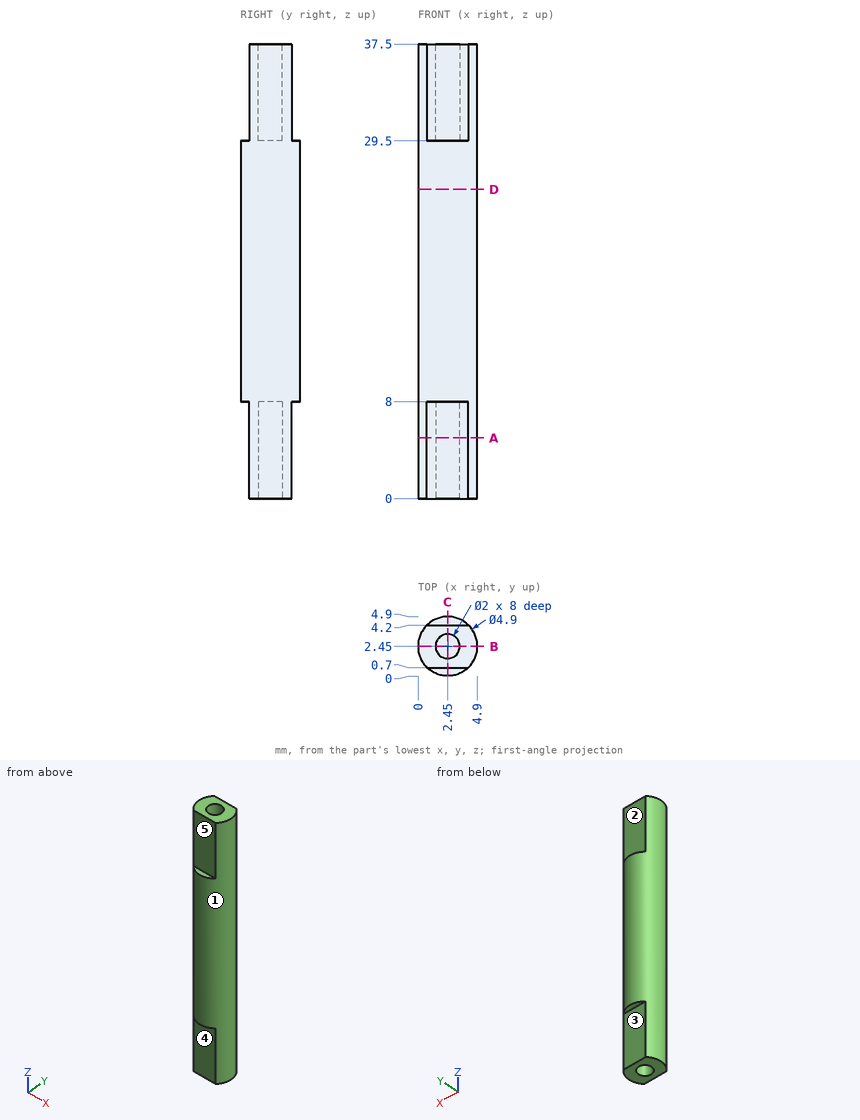
Geometry: see drawing. Coordinates: mm, zero at the bounding-box minimum. A direction names the side the tool comes from. Give positions to 0.01 mm unless a question says otherwise; leave off trailing zeros. Loops run counter-clockwise (first coordinate to the right, second up) from the corner with the lowest first, then second, coordinate; pieces in that order, holes last. Notation, with made-up numbers: (-10, 15) - (23, 15) arc R8 cw to (23, 21) - close; hole circle Ø9 at (7.25, 12). An arc over 180 degrees is marked (long way). Use CSV: the item, a comma, the result in double quotes. Start each with the question number.
1. Reachability of the marked faces 1, 2, 3, 4 and 5 from +Z, -Z, +X, -X, +Y, -Y: full face, straight path, thin tool, end or side. Return the list, or none.
2. Section C-C (x = 2.45). Output: boundary loops of the cut face in (y, z).
3. Ray query, L1, parallel to Y at x = 2.45, z = 6; L2, parallel to Z at x = 2.5, y = 2.2; L3, parallel to Y at x = 1.35, z = 2.5. Return the intervals inside material, ascending.
4. Section B-B (y = 2.45). Output: boundary loops of the cut face in (x, z), then the cut area to 3 significant figures.
5. Section A-A (z = 5). Output: boundary loops of the cut face in (x, y), then the cut area to 3 significant figures.
6. Pin query (flat end, axial travel): pin 1 (1.8 mm diameter, centred on x = 2.45, y = 2.45, fed in from +Z); pin 2 (2.5 mm diameter, centred on x = 2, z = 34, fed in from -Y); pin 3 (1 mm diameter, centred on x = 3, z = 35, fed in from +Y). Return the tip coordinate at first contact, or that it passes through.
7. Section D-D (z = 25.5). Output: boundary loops of the cut face in (x, y).
Response:
1,face 1,"+Z, -Z"
1,face 2,"+Z, +X, -X, +Y"
1,face 3,"-Z, +X, -X, +Y"
1,face 4,"-Z, +X, -X, -Y"
1,face 5,"+Z, +X, -X, -Y"
2,outline,"(0, 8) - (0.7, 8) - (0.7, 0) - (1.45, 0) - (1.45, 8) - (3.45, 8) - (3.45, 0) - (4.2, 0) - (4.2, 8) - (4.9, 8) - (4.9, 29.5) - (4.2, 29.5) - (4.2, 37.5) - (3.45, 37.5) - (3.45, 29.5) - (1.45, 29.5) - (1.45, 37.5) - (0.7, 37.5) - (0.7, 29.5) - (0, 29.5) - close"
3,L1,"0.7 to 1.45, 3.45 to 4.2"
3,L2,"8 to 29.5"
3,L3,"0.7 to 4.2"
4,outline,"(0, 0) - (1.45, 0) - (1.45, 8) - (3.45, 8) - (3.45, 0) - (4.9, 0) - (4.9, 37.5) - (3.45, 37.5) - (3.45, 29.5) - (1.45, 29.5) - (1.45, 37.5) - (0, 37.5) - close"
4,area,"152 mm²"
5,outline,"(0.74, 0.7) - (4.16, 0.7) arc R2.45 ccw to (4.16, 4.2) - (0.74, 4.2) arc R2.45 ccw to start; hole circle Ø2 at (2.45, 2.45)"
5,area,"12.4 mm²"
6,pin 1,"z = 29.5"
6,pin 2,"y = 0.7"
6,pin 3,"y = 4.2"
7,outline,"circle Ø4.9 at (2.45, 2.45)"
